Here's how the part is built. I have some questions about the finished solid (model axes, mm). A direction names the side the tool comes from. Round coordinates to 2 decimals unless told otherwise and drop trailing zeros. Loops run counter-clockwise (first coordinate to the right, second up) from the corner with the lowest first, then second, coordinate; pieces in that order, holes last. Notation, with made-up numbers: M 33,-9 L 48,-9 A27 ccw 48,21 Z; hole C 88.5,32.5 d5. An arc over 180 degrees is marked long. Answer as a JSON object with one key per item and string values.
from build123d import *

# Parameters (mm, degrees)
SKETCH1_W               = 127
SKETCH1_H               = 127
BOSS_EXTRUDE1_DEPTH     = 127
SKETCH2_W               = 76.2
SKETCH2_H               = 76.2
CUT_EXTRUDE1_DEPTH      = 1
CUT_EXTRUDE1_DEPTH_BACK = 128
FILLET3_R               = 6.35


with BuildPart() as part:
    # Sketch1 → Boss-Extrude1 (new body)
    with BuildSketch(Plane(origin=(0, 0, 0), x_dir=(1, 0, 0), z_dir=(0, 1, 0))):
        Rectangle(SKETCH1_W, SKETCH1_H)
    extrude(amount=BOSS_EXTRUDE1_DEPTH)

    # Sketch2 → Cut-Extrude1 (cut, two sides)
    with BuildSketch(Plane(origin=(0, 127, 0), x_dir=(1, 0, 0), z_dir=(0, 1, 0))) as cut_extrude1_sk:
        Rectangle(SKETCH2_W, SKETCH2_H)
    extrude(amount=CUT_EXTRUDE1_DEPTH, mode=Mode.SUBTRACT)
    extrude(cut_extrude1_sk.sketch, amount=-CUT_EXTRUDE1_DEPTH_BACK, mode=Mode.SUBTRACT)

    # Fillet3
    fillet3_edges = [part.edges().sort_by_distance(p)[0] for p in [
        (63.5, 127, 0),
        (0, 127, 63.5),
        (38.1, 127, 0),
        (38.1, 0, 0),
        (0, 127, 38.1),
        (0, 0, 38.1),
        (-38.1, 127, 0),
        (-38.1, 0, 0),
        (0, 127, -38.1),
        (0, 0, -38.1),
        (-63.5, 127, 0),
        (0, 0, 63.5),
        (63.5, 0, 0),
        (0, 0, -63.5),
        (-63.5, 0, 0),
        (0, 127, -63.5),
    ]]
    fillet(fillet3_edges, radius=FILLET3_R)


solid = part.part
Item 1: Please list where these lines run through material, in increasing order: probe 1 along X at (y, z) = (115.5, -31); probe 2 along Y at (x, z) = (6.5, -41). Write a range as from..to.
Resolved:
{"probe 1": "-63.5..-38.1, 38.1..63.5", "probe 2": "1.02..125.98"}
Item 2: I want a section at A-A, the plane z = -27. Please give me the cut outline in (x, y).
Resolved:
{"outline": "M -63.5,6.35 A6.35 ccw -57.15,0 L -44.45,0 A6.35 ccw -38.1,6.35 L -38.1,120.65 A6.35 ccw -44.45,127 L -57.15,127 A6.35 ccw -63.5,120.65 Z; M 38.1,6.35 A6.35 ccw 44.45,0 L 57.15,0 A6.35 ccw 63.5,6.35 L 63.5,120.65 A6.35 ccw 57.15,127 L 44.45,127 A6.35 ccw 38.1,120.65 Z"}
Item 3: I'm going to push flat-ended pins straight in: pin 1 Ø6 at (x, z) = (-40, -34.5) entering from +Y; pin 2 Ø2 at (x, z) = (-42, -25) entering from -Y. Where does each tip first touch, or does it pass through?
Resolved:
{"pin 1": "y = 126.83", "pin 2": "y = 0.17"}
Item 4: I want a section at C-C, the plane y = 96. Please give me the cut outline in (x, z), then the cut area to 3 significant figures.
Resolved:
{"outline": "M -63.5,-63.5 L 63.5,-63.5 L 63.5,63.5 L -63.5,63.5 Z; hole M -38.1,-38.1 L 38.1,-38.1 L 38.1,38.1 L -38.1,38.1 Z", "area": "10,300 mm²"}
Item 5: On a 3-axis mill with a long thin cutter (end or side, diameter ignored), from which of +Z, -Z, +X, -X, +Y, -Y can I reach the whole of each face in a straight line? I mean faces 1 (the face through (0.89, 125.09, 61.69)), 2 (the face through (-1, 64, -38.1)), 3 (the face through (0.62, 125.19, 40.01)), 4 (the face through (0.62, 1.81, 40.01)). Say none if no direction works.
Resolved:
{"face 1": "+Z, +X, -X, +Y", "face 2": "+Y, -Y", "face 3": "+Y", "face 4": "-Y"}
Item 6: I want a section at B-B, the plane x = -22.5. Please give me the cut outline in (y, z), then the cut area to 3 significant figures.
Resolved:
{"outline": "M 0,-57.15 A6.35 ccw 6.35,-63.5 L 120.65,-63.5 A6.35 ccw 127,-57.15 L 127,-44.45 A6.35 ccw 120.65,-38.1 L 6.35,-38.1 A6.35 ccw 0,-44.45 Z; M 0,44.45 A6.35 ccw 6.35,38.1 L 120.65,38.1 A6.35 ccw 127,44.45 L 127,57.15 A6.35 ccw 120.65,63.5 L 6.35,63.5 A6.35 ccw 0,57.15 Z", "area": "6,380 mm²"}
Item 7: If we mould it in two halves opening along Z, with no side actions, what happens to faces 5 (the face through (61.59, 125.19, -0.89)), 6 (the face through (0.89, 1.91, -61.69)), 7 (the face through (-1, 63, 63.5)), 8 (the face through (0.62, 125.19, -40.01))? For each: pulls with the +Z half, pulls with the -Z half, needs draft (parallel to the pull), parting line crosses it, or undercut.
Resolved:
{"face 5": "needs draft", "face 6": "pulls with the -Z half", "face 7": "pulls with the +Z half", "face 8": "undercut"}
